Check sheet for the modelled part. Datum: model origin and axes. Units: mm. Face numbers are marked on the shaded views. A direction names the side the tool comes from. Coordinates: 2 decimals unless noted, no trailing zeros. Loops run counter-clockwise (first coordinate to the right, second up) from the corner with the lowest first, then second, coordinate; pieces in that order, holes last. Notation, with made-up numbers: (45, 55.5) -> (53, 55.5) arc R22 cw to (53, 66.5) -> close; hole circle Ø10 at (9.5, -22). An arc over 180 degrees is marked (long way). Use CSV: the item, a comma, the result in double quotes. Start each with the question number.
1. Sectioned sample at A-A, the plane z = -27. Record the cut outline in (x, y).
2. Release check for a two-part mould opening along X. For the marked faces 3, 4, 5 and 6 record: pulls with the +X half, pulls with the -X half, needs draft (parallel to the pull), parting line crosses it, or undercut.
3. Thickness scan on L1, parallel to Z at x = 2, y = -26; L2, parallel to X at y = -53.5, z = 31.5; L3, parallel to X at y = -37.5, z = 53.5. Record the ranges inside material, lowest first.
4. Sectioned sample at B-B, the plane y = -54.5. Count the separate pieces of the cut face and the enclosed holes in it, and give its area (3 significant figures).
5. Set-up check for the marked faces 1 and 2: record each of +Z, -Z, +X, -X, +Y, -Y from which the full face is reachable in a straight line by a thin tool's end or side.
6. Gauge pin test, flat ends, axial feed: pin 1 (7 mm diameter, centred on x = 24.84, z = 30.93, fed in from +Y); pin 2 (9 mm diameter, centred on x = 1.5, z = 87.26, fed in from -Y); pin 3 (1.5 mm diameter, centred on y = -47.5, z = -29, fed in from -X); pin 4 (1.5 mm diameter, centred on x = -29, y = -48, fed in from +Z). Record the tip position at first contact, or that the pin passes through.
```python
from build123d import *

# Parameters (mm, degrees)
F0_R     = 4
F0_R_2   = 26.5
F1_DEPTH = 60
F2_SIZE  = 1
F3_SIZE  = 2
F4_SIZE2 = 29.8564064606
F4_SIZE  = 8
F6_D     = 8.5
F6_DEPTH = 25
F6_TIP   = 2.5536576309


with BuildPart() as f1:
    # F0 (on Front) → F1 (new body)
    with BuildSketch(Plane.XZ):
        with BuildLine():
            Line((-45.9991587698, 54.2627746064), (-45.9991587698, -58.2372253936))
            Line((-45.9991587698, -58.2372253936), (49.0008412302, -58.2372253936))
            Line((49.0008412302, -58.2372253936), (49.0008412302, 54.2627746064))
            ThreePointArc((49.0008412302, 54.2627746064), (1.5008412302, 101.7627746064), (-45.9991587698, 54.2627746064))
        make_face()
        with BuildLine():
            ThreePointArc((-30.9991587698, -4.7372253936), (-27.3379935347, 4.1016093712), (-18.4991587698, 7.7627746064))
            Line((-18.4991587698, 7.7627746064), (21.5008412302, 7.7627746064))
            ThreePointArc((21.5008412302, 7.7627746064), (30.339675995, 4.1016093712), (34.0008412302, -4.7372253936))
            Line((34.0008412302, -4.7372253936), (34.0008412302, -30.7372253936))
            ThreePointArc((34.0008412302, -30.7372253936), (30.339675995, -39.5760601585), (21.5008412302, -43.2372253936))
            Line((21.5008412302, -43.2372253936), (-18.4991587698, -43.2372253936))
            ThreePointArc((-18.4991587698, -43.2372253936), (-27.3379935347, -39.5760601585), (-30.9991587698, -30.7372253936))
            Line((-30.9991587698, -30.7372253936), (-30.9991587698, -4.7372253936))
        make_face(mode=Mode.SUBTRACT)
        with Locations((1.5008412302, 21.2627746064)):
            Circle(F0_R, mode=Mode.SUBTRACT)
        with Locations((-31.4991587698, 54.2627746064)):
            Circle(F0_R, mode=Mode.SUBTRACT)
        with Locations((-21.833682549, 30.9282508272)):
            Circle(F0_R, mode=Mode.SUBTRACT)
        with Locations((1.5008412302, 54.2627746064)):
            Circle(F0_R_2, mode=Mode.SUBTRACT)
        with Locations((-21.833682549, 77.5972983855)):
            Circle(F0_R, mode=Mode.SUBTRACT)
        with Locations((1.5008412302, 87.2627746064)):
            Circle(F0_R, mode=Mode.SUBTRACT)
        with Locations((24.8353650093, 30.9282508272)):
            Circle(F0_R, mode=Mode.SUBTRACT)
        with Locations((34.5008412302, 54.2627746064)):
            Circle(F0_R, mode=Mode.SUBTRACT)
        with Locations((24.8353650093, 77.5972983855)):
            Circle(F0_R, mode=Mode.SUBTRACT)
    extrude(amount=F1_DEPTH)

    # F2
    f2_edges = [f1.edges().sort_by_distance(p)[0] for p in [
        (-35.499159, -60, 54.262775),
        (-25.833683, -60, 77.597298),
        (-2.499159, -60, 87.262775),
        (20.835365, -60, 77.597298),
        (30.500841, -60, 54.262775),
        (20.835365, -60, 30.928251),
        (-2.499159, -60, 21.262775),
        (-25.833683, -60, 30.928251),
    ]]
    chamfer(f2_edges, length=F2_SIZE)

    # F3
    f3_edges = [f1.edges().sort_by_distance(p)[0] for p in [
        (1.500841, -60, 7.762775),
    ]]
    chamfer(f3_edges, length=F3_SIZE)

    # F4
    f4_edges = [f1.edges().sort_by_distance(p)[0] for p in [
        (1.500841, -60, 101.762775),
    ]]
    f4_side = f1.faces().sort_by_distance((1.500841, -60, 11.623554))[0]
    chamfer(f4_edges, length=F4_SIZE, length2=F4_SIZE2, reference=f4_side)

    # F6
    with Locations(Plane(origin=(0, 0, -58.2372253936), x_dir=(1, 0, 0), z_dir=(0, 0, -1))):
        with Locations((-35.9991587698, 25), (39.0008412302, 25)):
            Hole(F6_D / 2, depth=F6_DEPTH)
            with Locations((0, 0, -(F6_DEPTH + F6_TIP / 2))):  # 118° drill point
                Cone(0, F6_D / 2, F6_TIP, mode=Mode.SUBTRACT)


solid = f1.part
```
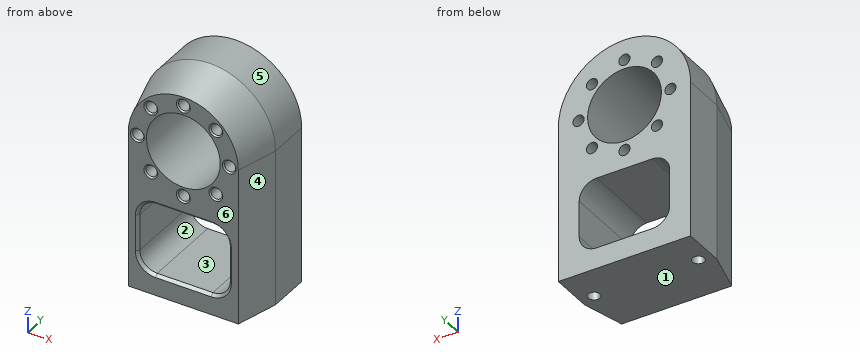
Completed:
1,outline,"(-46, -30.14) -> (-38, -60) -> (-33, -60) -> (-31, -58) -> (-31, 0) -> (-46, 0) -> close; (34, -58) -> (36, -60) -> (41, -60) -> (49, -30.14) -> (49, 0) -> (34, 0) -> close"
2,face 3,"undercut"
2,face 4,"pulls with the +X half"
2,face 5,"parting line crosses it"
2,face 6,"needs draft"
3,L1,"-58.24 to -43.24, 7.76 to 17.29, 25.23 to 27.77, 80.76 to 83.29, 91.23 to 101.76"
3,L2,"-39.74 to -25.79, -17.87 to -12.07, 15.07 to 20.88, 28.79 to 42.74"
3,L3,"-44.03 to -35.43, -27.57 to -24.99, 27.99 to 30.57, 38.43 to 47.03"
4,separate pieces,"1"
4,enclosed holes,"10"
4,area,"6,070 mm²"
5,face 1,"-Z, +X, -X, +Y, -Y"
5,face 2,"+Y, -Y"
6,pin 1,"through"
6,pin 2,"y = -59.5"
6,pin 3,"x = -41.55"
6,pin 4,"z = 84.97"
